```python
from build123d import *

# Parameters (mm, degrees)
CROQUIS1_R              = 2.495
SALIENTE_EXTRUIR1_DEPTH = 6.9
REDONDEO1_R             = 0.1
CROQUIS2_R              = 0.75
CORTAR_EXTRUIR1_DEPTH   = 3


with BuildPart() as part:
    # Croquis1 → Saliente-Extruir1 (new body)
    with BuildSketch(Plane(origin=(0, 0, 0), x_dir=(1, 0, 0), z_dir=(0, 1, 0))):
        Circle(CROQUIS1_R)
    extrude(amount=SALIENTE_EXTRUIR1_DEPTH)

    # Redondeo1
    redondeo1_edges = [part.edges().sort_by_distance(p)[0] for p in [
        (-2.495, 0, 0),
        (-2.495, 6.9, 0),
    ]]
    fillet(redondeo1_edges, radius=REDONDEO1_R)

    # Croquis2 → Cortar-Extruir1 (cut)
    with BuildSketch(Plane(origin=(0, 6.9, 0), x_dir=(1, 0, 0), z_dir=(0, 1, 0))):
        Circle(CROQUIS2_R)
    extrude(amount=-CORTAR_EXTRUIR1_DEPTH, mode=Mode.SUBTRACT)


solid = part.part
```
Part model, mm, in its own coordinate system. A direction names the side the tool comes from. Round coordinates to 2 decimals unless told otherwise and drop trailing zeros. Loops run counter-clockwise (first coordinate to the right, second up) from the corner with the lowest first, then second, coordinate; pieces in that order, holes last. Notation, with made-up numbers: (50.25, 75) -> (62.25, 75) arc R16 cw to (62.25, 92) -> close; hole circle Ø11 at (53, -29.5). An arc over 180 degrees is marked (long way). Use CSV: the item, a comma, the result in double quotes. Start each with the question number.
1) Wall check: L1, parallel to Z at x = 0, y = 6.05 (3 decimals); L2, parallel to Z at x = 0.45, y = 4.75. Give the ranges that are in metal, low to high. Write a range as [from, to].
2) Cut at A-A, the plane z = 0. Write the cut outline in (x, y) (3 decimals), plus the area to 3 significant figures.
3) Pull direction X, two halves, no side cores. Call faces 3 (the cylindrical face through (-0.325, 3.403, -2.474)), 4 (the flat face through (0, 3.9, 0)), 5 (the flat face through (-1, 6.9, 0)): +X half, -X half, draft (parallel to the pull), parting line (faces both ways), or undercut.
4) Cut at D-D, the plane y = 4. Write the cut outline in (x, z) (3 decimals), plus the area to 3 significant figures.
5) Drop a flat-ended pin along its axis: P1, Ø0.8, axis at x = 0, z = 0, coming from the +Y side. Give the stop position or say it passes through.
6) Which spindle directions (+Z, -Z, +X, -X, +Y, -Y) get a long thin tool onto all of the face, cutting with end or side? Do faces 1 (the flat face through (0, 0, 0)), 2 (the cylindrical face through (-0.75, 5.42, -0.03)). Say none if no direction does.
7) Cut at B-B, the plane x = 0. Write the cut outline in (y, z) (3 decimals).
8) Cut at C-C, the plane y = 1. Write the cut outline in (x, z) (3 decimals).
Determined:
1,L1,"z = [-2.495, -0.75], [0.75, 2.495]"
1,L2,"z = [-2.45, -0.6], [0.6, 2.45]"
2,outline,"(-2.495, 0.1) arc R0.1 ccw to (-2.395, 0) -> (2.395, 0) arc R0.1 ccw to (2.495, 0.1) -> (2.495, 6.8) arc R0.1 ccw to (2.395, 6.9) -> (0.75, 6.9) -> (0.75, 3.9) -> (-0.75, 3.9) -> (-0.75, 6.9) -> (-2.395, 6.9) arc R0.1 ccw to (-2.495, 6.8) -> close"
2,area,"29.9 mm2"
3,face 3,"parting line"
3,face 4,"undercut"
3,face 5,"draft"
4,outline,"circle Ø4.99 at (0, 0); hole circle Ø1.5 at (0, 0)"
4,area,"17.8 mm2"
5,P1,"stops at y = 3.9"
6,face 1,"+Z, -Z, +X, -X, -Y"
6,face 2,"+Y"
7,outline,"(0, -2.395) arc R0.1 ccw to (0.1, -2.495) -> (6.8, -2.495) arc R0.1 ccw to (6.9, -2.395) -> (6.9, -0.75) -> (3.9, -0.75) -> (3.9, 0.75) -> (6.9, 0.75) -> (6.9, 2.395) arc R0.1 ccw to (6.8, 2.495) -> (0.1, 2.495) arc R0.1 ccw to (0, 2.395) -> close"
8,outline,"circle Ø4.99 at (0, 0)"
